The listing builds one solid part. Answer for the finished solid, in the listing's coordinates (mm). A direction names the side the tool comes from. Give positions to 0.01 mm unless a question says otherwise; leave off trailing zeros. Loops run counter-clockwise (first coordinate to the right, second up) from the corner with the lowest first, then second, coordinate; pieces in that order, holes last. Notation, with made-up numbers: (48, -6) - (61, -6) arc R21 ccw to (61, 8) - close; hole circle Ø1 at (25, -38.5). An arc over 180 degrees is marked (long way). Write item = value, one per line. Start each with the question number.
1) Consider probe 1 along Z at (x, y) = (7, 0); probe 2 along Z at (x, y) = (-10, 17); probe 3 along Z at (x, y) = (-16.5, -0.5). Determine where each line is inside the solid, lowest interval first.
2) The part is cut by section C-C on z = 90. Write down the section's boundary in (x, y), plus the area to 3 significant figures.
3) The mould has two halves that part along Y. Classify faces 6 (the cylindrical face through (19.076, 6.007, 1.61)), 7 (the cylindrical face through (2.255, -2.628, 98.346)), 8 (the flat face through (-15, -9, -90)): +Y half, -Y half, draft (parallel to the pull), parting line (faces both ways), or undercut.
4) Which of the six approach directions +Z, -Z, +X, -X, +Y, -Y give full straight-line access (tool end or side, diameter ignored) to faces 1 (the flat face through (2, 0, -115)), 2 (the flat face through (2, 0, 115)), 3 (the flat face through (0, 17, 50)), 4 (the flat face through (0, -17, -50)), 5 (the flat face through (-15, -9, 90))?
5) Flat-ended cylindrical pins translate along their axes: P1, Ø10, axis at y = -6, z = -46.5, coming from the +X side (3 decimals); P2, Ø4, axis at y = 5, z = 33, coming from the -X side; P3, Ø6, axis at y = -3.5, z = 82, coming from the -X side. Find the tip coordinate at first contact, or state that the pin passes through.
6) The part is cut by section B-B on x = 0. Write down the section's boundary in (y, z), plus the area to 3 significant figures.
7) The part is cut by section A-A on y = 0. Write down the section's boundary in (x, z), plus the area to 4 significant figures.
8) The part is cut by section D-D on y = 11. Write down the section's boundary in (x, z).
from build123d import *

# Parameters (mm, degrees)
SKETCH_1_R           = 20
EXTRUDE_1_DEPTH      = 115
CUT_EXTRUDE_START    = -65
SKETCH_2_OUTSIDE_W   = 89.37
SKETCH_2_OUTSIDE_H   = 89.37
SKETCH_2_OUTSIDE_W_2 = 80.530626202
SKETCH_2_OUTSIDE_H_2 = 30
CUT_EXTRUDE_1_DEPTH  = 15.2
CUT_EXTRUDE_2_DEPTH  = 50


with BuildPart() as part:
    # 草图1 → 凸台-拉伸1 (new, symmetric)
    with BuildSketch(Plane.XY):
        Circle(SKETCH_1_R)
    extrude(amount=EXTRUDE_1_DEPTH, both=True)

    # 草图2 outside → 切除-拉伸1 (cut)
    with BuildSketch(Plane.XY.offset(115).offset(CUT_EXTRUDE_START)):
        Rectangle(SKETCH_2_OUTSIDE_W, SKETCH_2_OUTSIDE_H)
        Rectangle(SKETCH_2_OUTSIDE_W_2, SKETCH_2_OUTSIDE_H_2, mode=Mode.SUBTRACT)
    cut_extrude_1 = extrude(amount=-CUT_EXTRUDE_1_DEPTH, mode=Mode.SUBTRACT)

    # 草图3 → 切除-拉伸2 (cut)
    with BuildSketch(Plane.XY.offset(115)):
        Polygon((-15, -119.751298217), (-15, -13.228756555), (-15, 13.228756555), (-15, 119.751298217), (-228.045083324, 119.751298217), (-228.045083324, -119.751298217), align=None)
    cut_extrude_2 = extrude(amount=-CUT_EXTRUDE_2_DEPTH, mode=Mode.SUBTRACT)

    # 草图4 → M20 螺纹孔1 (revolve, cut)
    with BuildSketch(Plane(origin=(-15, 0, 90), x_dir=(0, 0, 1), z_dir=(0, 1, 0))):
        Polygon((0, 0), (0, 52.757530416), (8.75, 47.5), (8.75, 0), align=None)
    hole_wizard_m20_1 = revolve(axis=Axis((-21.35, 0, 90), (1, 0, 0)), mode=Mode.SUBTRACT)

    # 镜向1: 切除-拉伸1, 切除-拉伸2, M20 螺纹孔1 across plane
    add(cut_extrude_1.mirror(Plane.XY), mode=Mode.SUBTRACT)
    add(cut_extrude_2.mirror(Plane.XY), mode=Mode.SUBTRACT)
    add(hole_wizard_m20_1.mirror(Plane.XY), mode=Mode.SUBTRACT)


solid = part.part
Answer below:
q1.probe_1 = -115 to -98.75, -81.25 to 81.25, 98.75 to 115
q1.probe_2 = -115 to -50, -34.8 to 34.8, 50 to 115
q1.probe_3 = -65 to 65
q2.outline = (-15, -13.23) arc R20 ccw to (17.98, -8.75) - (-15, -8.75) - close; (-15, 8.75) - (17.98, 8.75) arc R20 ccw to (-15, 13.23) - close
q2.area = 565 mm2
q3.face_6 = parting line
q3.face_7 = undercut
q3.face_8 = draft
q4.face_1 = -Z, +X, -X, +Y, -Y
q4.face_2 = +Z, +X, -X, +Y, -Y
q4.face_3 = +X, -X, +Y
q4.face_4 = +X, -X, -Y
q4.face_5 = +Z, -X, +Y, -Y
q5.P1 = 19.975
q5.P2 = -19.77
q5.P3 = -15
q6.outline = (-20, -115) - (20, -115) - (20, -50) - (15, -50) - (15, -34.8) - (20, -34.8) - (20, 34.8) - (15, 34.8) - (15, 50) - (20, 50) - (20, 115) - (-20, 115) - (-20, 50) - (-15, 50) - (-15, 34.8) - (-20, 34.8) - (-20, -34.8) - (-15, -34.8) - (-15, -50) - (-20, -50) - close; hole circle Ø17.5 at (0, -90); hole circle Ø17.5 at (0, 90)
q6.area = 8,410 mm2
q7.outline = (-20, -65) - (-15, -65) - (-15, -81.25) - (20, -81.25) - (20, 81.25) - (-15, 81.25) - (-15, 65) - (-20, 65) - close; (-15, -115) - (20, -115) - (20, -98.75) - (-15, -98.75) - close; (-15, 98.75) - (20, 98.75) - (20, 115) - (-15, 115) - close
q7.area = 7,475 mm2
q8.outline = (-16.7, -65) - (-15, -65) - (-15, -115) - (16.7, -115) - (16.7, 115) - (-15, 115) - (-15, 65) - (-16.7, 65) - close
